from build123d import *
from build123d import SkipClean  # not in build123d's __all__

# Parameters (mm, degrees)
F0_W      = 4
F0_H      = 20
F1_DEPTH  = 4
F2_W      = 5.5
F2_H      = 20
F3_DEPTH  = 2
F4_W      = 5
F4_H      = 20
F5_DEPTH  = 10
F6_W      = 5
F6_H      = 20
F7_DEPTH  = 150
F8_W      = 5
F8_H      = 5
F9_DEPTH  = 140
F10_W     = 5
F10_H     = 163
F11_DEPTH = 50
F12_W     = 9.4903359083
F12_H     = 16
F13_DEPTH = 20
F14_W     = 15.6903359083
F14_H     = 16
F15_DEPTH = 30
F17_DEPTH = 16
F19_DEPTH = 5.5
F21_DEPTH = 4


with BuildPart() as f1:
    # F0 (on Top) → F1 (new body)
    with BuildSketch(Plane.XY):
        with Locations((2, 10)):
            Rectangle(F0_W, F0_H)
    extrude(amount=F1_DEPTH)

    # F2 (on Top) → F3 (join)
    with BuildSketch(Plane.XY):
        with Locations((6.75, 10)):
            Rectangle(F2_W, F2_H)
    extrude(amount=F3_DEPTH)

    # F4 (on Top) → F5 (join)
    with BuildSketch(Plane.XY):
        with Locations((12, 10)):
            Rectangle(F4_W, F4_H)
    extrude(amount=F5_DEPTH)

    # F6 (on Top) → F7 (join)
    with BuildSketch(Plane.XY):
        with Locations((17, 10)):
            Rectangle(F6_W, F6_H)
        Polygon((24.8, 0), (19.5, 20), (19.5, 0), align=None)
    extrude(amount=F7_DEPTH)

    # F8 (on face) → F9 (join)
    with BuildSketch(Plane.XY.offset(10)):
        with Locations((12, 17.5)):
            Rectangle(F8_W, F8_H)
        with Locations((12, 2.5)):
            Rectangle(F8_W, F8_H)
    extrude(amount=F9_DEPTH)

    # F10 (on face) → F11 (join)
    with BuildSketch(Plane(origin=(23.17269733, 6.1407647925, 0), x_dir=(-0.2561582385, 0.9666348622, 0), z_dir=(0.9666348622, 0.2561582385, 0))):
        with Locations((-3.8527243145, 81.5)):
            Rectangle(F10_W, F10_H)
    extrude(amount=F11_DEPTH)

    # F12 (on face) → F13 (join)
    with BuildSketch(Plane(origin=(23.17269733, 6.1407647925, 0), x_dir=(-0.2561582385, 0.9666348622, 0), z_dir=(0.9666348622, 0.2561582385, 0))):
        Polygon((14.3376115938, 0), (14.3376115938, 150), (8.1376115938, 150), (8.1376115938, 16), (8.1376115938, 0), align=None)
        with Locations((3.3924436397, 8)):
            Rectangle(F12_W, F12_H)
    extrude(amount=F13_DEPTH)

    # F14 (on face) → F15 (join)
    with BuildSketch(Plane(origin=(42.5053945744, 11.2639295622, 0), x_dir=(-0.2561582385, 0.9666348622, 0), z_dir=(0.9666348622, 0.2561582385, 0))):
        with Locations((6.4924436397, 8)):
            Rectangle(F14_W, F14_H)
    extrude(amount=F15_DEPTH)

    # F16 (on face) → F17 (cut)
    with BuildSketch(Plane.XY.offset(16)):
        Polygon((67.8317431109, 32.8079119244), (38.8326972444, 25.1231647698), (71.8509519185, 17.6410862355), align=None)
    extrude(amount=-F17_DEPTH, mode=Mode.SUBTRACT)

    # F18 (on face) → F19 (join)
    with BuildSketch(Plane.XY.offset(163)):
        Polygon((71.8509519185, 17.6410862355), (23.5192088076, 4.8331743111), (24.0315252845, 2.8999045867), (72.3632683954, 15.707816511), align=None)
    extrude(amount=F19_DEPTH)

    # F20 (on face) → F21 (join)
    with BuildSketch(Plane.XY.offset(168.5)):
        Polygon((71.8509515411, 17.6410861355), (23.5192088076, 4.8331743111), (24.287683523, 1.9332697244), (72.6194262566, 14.7411815488), align=None)
    with SkipClean():  # cleaning this boolean's faces spoils the solid; the shape is the same uncleaned
        extrude(amount=F21_DEPTH)


solid = f1.part
Model file for the job. Use its own axes, mm. A direction names the side the tool comes from. Give positions to 0.01 mm unless a question says otherwise; leave off trailing zeros. Write each loop counter-clockwise with the first axis right and the second up, starting at its lowest first coordinate (ties: lowest second). Pieces come first, ordered by that corner, then holes. Notation, with made-up numbers: (-32, 47.5) - (12, 47.5) arc R16 cw to (12, 74.5) - close; hole circle Ø4 at (20.5, -38). An arc over 180 degrees is marked (long way). Answer as CSV lines item,"result".
1. Band-saw the part on A-A (z = 123). Write the cut outline in (x, y).
Responses:
outline,"(9.5, 0) - (24.8, 0) - (73.13, 12.81) - (71.85, 17.64) - (23.52, 4.83) - (21.09, 14.01) - (40.42, 19.13) - (38.83, 25.12) - (19.5, 20) - (9.5, 20) - (9.5, 15) - (14.5, 15) - (14.5, 5) - (9.5, 5) - close"
2. Two-plate mould, pull along Y, no slides. Class faces 1 (the face through (0, 10, 2)), 2 (the face through (12, 10, 10)), 3 (the face through (18, 0, 74)): +Y half, -Y half, draft (parallel to the pull), parting line (faces both ways), or undercut.
Responses:
face 1,"draft"
face 2,"undercut"
face 3,"-Y half"
3. Band-saw the part on C-C (x = 51). Write the cut outline in (y, z).
Responses:
outline,"(6.94, 0) - (22.37, 0) - (22.37, 16) - (12.12, 16) - (12.12, 172.5) - (9.01, 172.5) - (9.01, 168.5) - (10.05, 168.5) - (10.05, 163) - (6.94, 163) - close"
4. Band-saw the part on D-D (x = 61.5). Write the cut outline in (y, z).
Responses:
outline,"(9.73, 0) - (19.99, 0) - (19.99, 16) - (14.9, 16) - (14.9, 172.5) - (11.79, 172.5) - (11.79, 168.5) - (12.83, 168.5) - (12.83, 163) - (9.73, 163) - close"
5. 3-axis set-ups, long thin cutter, end or side, ignore diameter. For faces 4 (the face through (7, 10, 2)), 5 (the face through (22.32, 9.36, 82.06)), 6 (the face through (14, 20, 74)), 7 (the face through (48, 8, 163)): which of +Z, -Z, +X, -X, +Y, -Y reach the whole face in a straight line?
Responses:
face 4,"+Z, +Y, -Y"
face 5,"+Z"
face 6,"+Z, -Z, -X, +Y"
face 7,"+X, -Y"
6. Drill centre lines: L1, parallel to Z at x = 34, y = 5.5; L2, parallel to Z at x = 15.5, y = 9.75; L3, parallel to Y at x = 25, z = 89.5. Where is each one in solid material? Low to high. Write a range as [from, to].
Responses:
L1,"z = [0, 163], [168.5, 172.5]"
L2,"z = [0, 150]"
L3,"y = [0.05, 5.23], [15.04, 21.46]"
7. Pin check, flat tips, straight feed: pin 1 (6 mm diameter, centred on x = 34.5, y = 10.5, fed in from +Z); pin 2 (12 mm diameter, centred on y = 19.5, z = 71.5, fed in from -X); pin 3 (10 mm diameter, centred on y = 18, z = 88, fed in from +X); pin 4 (3 mm diameter, centred on y = 9, z = 86.5, fed in from -X). Stop position of each tip, or through.
Responses:
pin 1,"stops at z = 172.5"
pin 2,"stops at x = 9.5"
pin 3,"stops at x = 73.08"
pin 4,"stops at x = 14.5"
8. Band-saw the part on B-B (x = 33). Write the cut outline in (y, z), and give its area (3 significant figures).
Responses:
outline,"(2.17, 0) - (23.58, 0) - (23.58, 150) - (17.16, 150) - (17.16, 16) - (7.35, 16) - (7.35, 172.5) - (4.24, 172.5) - (4.24, 168.5) - (5.28, 168.5) - (5.28, 163) - (2.17, 163) - close"
area,"1,990 mm2"
